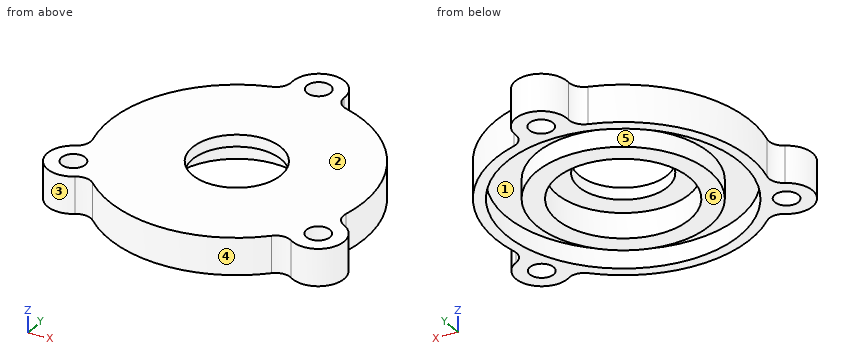
```python
from build123d import *

# Parameters (mm, degrees)
SKETCH_1_R          = 6
SKETCH_1_R_2        = 1.6
EXTRUDE_1_DEPTH     = 5
FILLET_1_R          = 2
SKETCH_3_R          = 15.8
SKETCH_3_R_2        = 11.7
CUT_EXTRUDE_1_DEPTH = 2.5
SKETCH_4_R          = 9
CUT_EXTRUDE_2_DEPTH = 3.4


with BuildPart() as part:
    # ｽｹｯﾁ1 → ﾎﾞｽ - 押し出し1 (new body)
    with BuildSketch(Plane.XY):
        with BuildLine():
            ThreePointArc((-3.021819699, 17.034042553), (-14.982239485, 8.65), (-16.26282343, -5.900048651))
            ThreePointArc((-16.26282343, -5.900048651), (-19.312366504, -11.15), (-13.24100373, -11.133993902))
            ThreePointArc((-13.24100373, -11.133993902), (0, -17.3), (13.24100373, -11.133993902))
            ThreePointArc((13.24100373, -11.133993902), (19.312366504, -11.15), (16.26282343, -5.900048651))
            ThreePointArc((16.26282343, -5.900048651), (14.982239485, 8.65), (3.021819699, 17.034042553))
            ThreePointArc((3.021819699, 17.034042553), (0, 22.3), (-3.021819699, 17.034042553))
        make_face()
        Circle(SKETCH_1_R, mode=Mode.SUBTRACT)
        with Locations((0, 18.8)):
            Circle(SKETCH_1_R_2, mode=Mode.SUBTRACT)
        with Locations((16.281277591, -9.4)):
            Circle(SKETCH_1_R_2, mode=Mode.SUBTRACT)
        with Locations((-16.281277591, -9.4)):
            Circle(SKETCH_1_R_2, mode=Mode.SUBTRACT)
    extrude(amount=EXTRUDE_1_DEPTH)

    # ﾌｨﾚｯﾄ1
    fillet_1_edges = [part.edges().sort_by_distance(p)[0] for p in [
        (16.26282343, -5.900048651, 2.5),
        (13.24100373, -11.133993902, 2.5),
        (-13.24100373, -11.133993902, 2.5),
        (-16.26282343, -5.900048651, 2.5),
        (-3.021819699, 17.034042553, 2.5),
        (3.021819699, 17.034042553, 2.5),
    ]]
    fillet(fillet_1_edges, radius=FILLET_1_R)

    # ｽｹｯﾁ3 → ｶｯﾄ - 押し出し1 (cut)
    with BuildSketch(Plane(origin=(0, 0, 0), x_dir=(-1, 0, 0), z_dir=(0, 0, -1))):
        Circle(SKETCH_3_R)
        Circle(SKETCH_3_R_2, mode=Mode.SUBTRACT)
    extrude(amount=-CUT_EXTRUDE_1_DEPTH, mode=Mode.SUBTRACT)

    # ｽｹｯﾁ4 → ｶｯﾄ - 押し出し2 (cut)
    with BuildSketch(Plane(origin=(0, 0, 0), x_dir=(-1, 0, 0), z_dir=(0, 0, -1))):
        Circle(SKETCH_4_R)
    extrude(amount=-CUT_EXTRUDE_2_DEPTH, mode=Mode.SUBTRACT)


solid = part.part
```
Source: CAD feature listing. Evaluate the final solid. Frame: model axes, mm. Face numbers are marked on the shaded views. A direction names the side the tool comes from. Coordinates: 2 decimals unless noted, no trailing zeros. Order: outer loops, then holes, each group sorted by start corner. A loop starts at its lowest first (then second) coordinate and runs counter-clockwise, first axis right, second up. Notation, with made-up numbers: (33, 1) - (69, 1) arc R27 cw to (69, 30) - close; hole circle Ø1 at (59.5, 83.5). An arc over 180 degrees is marked (long way). One line per item, written item: value.
1) Reachability of the marked faces 5 and 6 from +Z, -Z, +X, -X, +Y, -Y: full face, straight path, thin tool, end or side. Return the list, or none.
Computed values:
face 5: -Z
face 6: -Z, +X, -X, +Y, -Y
2) Cut plane C-C on z = 1.2. State how many separate pieces and enclosed holes the cut face has, plus the area to 3 significant figures.
Computed values:
separate pieces: 2
enclosed holes: 5
area: 402 mm^2
3) Cut plane A-A on y = 0. Output: boundary loops of the cut face in (x, z), plus the area to 3 significant figures.
Computed values:
outline: (-17.3, 0) - (-15.8, 0) - (-15.8, 2.5) - (-11.7, 2.5) - (-11.7, 0) - (-9, 0) - (-9, 3.4) - (-6, 3.4) - (-6, 5) - (-17.3, 5) - close; (6, 3.4) - (9, 3.4) - (9, 0) - (11.7, 0) - (11.7, 2.5) - (15.8, 2.5) - (15.8, 0) - (17.3, 0) - (17.3, 5) - (6, 5) - close
area: 72.1 mm^2
4) Cut plane B-B on x = 0. Output: boundary loops of the cut face in (y, z).
Computed values:
outline: (-17.3, 0) - (-15.8, 0) - (-15.8, 2.5) - (-11.7, 2.5) - (-11.7, 0) - (-9, 0) - (-9, 3.4) - (-6, 3.4) - (-6, 5) - (-17.3, 5) - close; (6, 3.4) - (9, 3.4) - (9, 0) - (11.7, 0) - (11.7, 2.5) - (15.8, 2.5) - (15.8, 0) - (17.2, 0) - (17.2, 5) - (6, 5) - close; (20.4, 0) - (22.3, 0) - (22.3, 5) - (20.4, 5) - close
5) Cut plane D-D on x = -7. Output: boundary loops of the cut face in (y, z), plus the area to 3 significant figures.
Computed values:
outline: (-15.82, 0) - (-14.16, 0) - (-14.16, 2.5) - (-9.37, 2.5) - (-9.37, 0) - (-5.66, 0) - (-5.66, 3.4) - (5.66, 3.4) - (5.66, 0) - (9.37, 0) - (9.37, 2.5) - (14.16, 2.5) - (14.16, 0) - (15.82, 0) - (15.82, 5) - (-15.82, 5) - close
area: 95.8 mm^2
6) Contact query for flat-ended pins moving along their axis: pin 1 (19 mm diameter, centred on x = 0, y = 0, fed in from -Z); pin 2 (3 mm diameter, centred on y = 2, z = 3.5, fed in from +X); pin 3 (3 mm diameter, centred on x = -6, z = 2, fed in from -Y); pin 4 (2 mm diameter, centred on x = -15, z = 0.5, fed in from +Y). Output: stop coordinate, or through.
Computed values:
pin 1: stops at z = 0
pin 2: stops at x = 17.29
pin 3: stops at y = -16.7
pin 4: stops at y = 10.16
7) Ray query, line 1 (Y direction, x = -3, z = 2.2); line 2 (X direction, y = -10.5, z = 1.8); line 3 (Y direction, x = 0, z = 1.75). Return the intervals inside material, ascending. Write a range as [from, to].
Computed values:
line 1: y = [-17.04, -15.51], [-11.31, -8.49], [8.49, 11.31], [15.51, 20.6]
line 2: x = [-19.6, -17.44], [-15.12, -11.81], [-5.16, 5.16], [11.81, 15.12], [17.44, 19.6]
line 3: y = [-17.3, -15.8], [-11.7, -9], [9, 11.7], [15.8, 17.2], [20.4, 22.3]
8) Mould query, pull axis Y, two halves, no side actions, for the marked faces 1, 2, 3 and 4. Classes: released by +Y, released by -Y, zero draft, split by the parting line, or undercut.
Computed values:
face 1: undercut
face 2: zero draft
face 3: split by the parting line
face 4: released by -Y
